Source: CAD feature listing. Evaluate the final solid. Frame: model axes, mm. A direction names the side the tool comes from. Coordinates: 2 decimals unless noted, no trailing zeros. Order: outer loops, then holes, each group sorted by start corner. A loop starts at its lowest first (then second) coordinate and runs counter-clockwise, first axis right, second up. Notation, with made-up numbers: (-26.75, -22.75) -> (-12.75, -22.75) arc R24 cw to (-12.75, -1.75) -> close; hole circle Ø4 at (0, 35.25). An arc over 180 degrees is marked (long way). Write item = value, one per line. Start each with the question number.
Item 1: Mould query, pull axis Y, two halves, no side actions, for faces 1 (the cylindrical face through (218, 2, 3)), 2 (the flat face through (0, 69, 3)), 3 (the cylindrical face through (8, 128, 3)). Classes: released by +Y, released by -Y, zero draft, split by the parting line, or undercut.
Item 2: Section query A-A (y = 84). Output: boundary loops of the cut face in (x, z).
Item 3: Set-up query: faces 4 (the cylindrical face through (9, 8, 3)), 5 (the flat face through (101, 3, 0)). Return all of +Z, -Z, +X, -X, +Y, -Y with unobstructed straight access to the full face (end or side cutting, diameter ignored); none if empty.
Item 4: Section query B-B (z = 4.8). Output: boundary loops of the cut face in (x, y), then the cut area to 3 significant figures.
Item 5: Section query C-C (x = 187.5). Output: boundary loops of the cut face in (y, z), then the cut area to 3 significant figures.
Item 6: Ray query, line 1 along Y through (x, z) = (14, 0.6); line 2 along X through (y, z) = (107.5, 4.8); line 3 along Y through (x, z) = (210, 0.9). Return the intervals inside material, ascending. Write a range as [from, to].
Autodesk Fusion 360 part; units mm, degrees
sketch "Esquisse1" plane through (0, 0, 0) normal (0, 0, 1) x (1, 0, 0)
  line L0 (5, 0) -> (214, 0)
  line L1 (219, 5) -> (219, 132)
  line L2 (214, 137) -> (5, 137)
  line L3 (0, 132) -> (0, 5)
  line L4 (12, 7) -> (207, 7)
  line L5 (212, 12) -> (212, 125)
  line L6 (207, 130) -> (12, 130)
  line L7 (7, 125) -> (7, 12)
  arc A0 (219, 132) -> (214, 137) centre (214, 132) ccw
  arc A1 (212, 125) -> (207, 130) centre (207, 125) ccw
  arc A2 (214, 0) -> (219, 5) centre (214, 5) ccw
  arc A3 (207, 7) -> (212, 12) centre (207, 12) ccw
  arc A4 (7, 12) -> (12, 7) centre (12, 12) ccw
  arc A5 (0, 5) -> (5, 0) centre (5, 5) ccw
  arc A6 (12, 130) -> (7, 125) centre (12, 125) ccw
  arc A7 (5, 137) -> (0, 132) centre (5, 132) ccw
  point P0 (219, 137)
  point P1 (0, 137)
  point P2 (7, 7)
  point P3 (212, 130)
  point P4 (7, 130)
  dimension "d1" = 219
  dimension "d2" = 205
  dimension "d3" = 7
  dimension "d4" = 123
  dimension "d5" = 7
  dimension "d6" = 137
  dimension "d7" = 5
  dimension "d8" = 5
  dimension "d9" = 5
  dimension "d10" = 5
  dimension "d11" = 5
  dimension "d12" = 5
  dimension "d13" = 5
  dimension "d14" = 5
extrude "Extrusion1" add sketch "Esquisse1" along normal blind 6
Computed:
q1.face_1 = released by -Y
q1.face_2 = zero draft
q1.face_3 = undercut
q2.outline = (0, 0) -> (7, 0) -> (7, 6) -> (0, 6) -> close; (212, 0) -> (219, 0) -> (219, 6) -> (212, 6) -> close
q3.face_4 = +Z, -Z
q3.face_5 = -Z, +X, -X, +Y, -Y
q4.outline = (0, 5) arc R5 ccw to (5, 0) -> (214, 0) arc R5 ccw to (219, 5) -> (219, 132) arc R5 ccw to (214, 137) -> (5, 137) arc R5 ccw to (0, 132) -> close; hole (7, 12) arc R5 ccw to (12, 7) -> (207, 7) arc R5 ccw to (212, 12) -> (212, 125) arc R5 ccw to (207, 130) -> (12, 130) arc R5 ccw to (7, 125) -> close
q4.area = 4,790 mm^2
q5.outline = (0, 0) -> (7, 0) -> (7, 6) -> (0, 6) -> close; (130, 0) -> (137, 0) -> (137, 6) -> (130, 6) -> close
q5.area = 84.0 mm^2
q6.line_1 = [0, 7], [130, 137]
q6.line_2 = [0, 7], [212, 219]
q6.line_3 = [0, 8], [129, 137]
